from build123d import *

# Parameters (mm, degrees)
F0_W     = 18.5
F0_H     = 6.9
F0_H_2   = 6.8
F1_DEPTH = 3.25
F3_DEPTH = 1.5
F4_R     = 5
F6_D     = 4.4
F8_D     = 4.4


with BuildPart() as f1:
    # F0 (on Top) → F1 (new body)
    with BuildSketch(Plane.XY):
        with BuildLine():
            Line((-14.6952698517, 19.7279642442), (-29.6952698517, 19.7279642442))
            Line((-29.6952698517, 19.7279642442), (-41.8622746435, 10.5594685057))
            ThreePointArc((-41.8622746435, 10.5594685057), (-43.1340644308, 9.1283890545), (-43.7536388636, 7.3168799651))
            Line((-43.7536388636, 7.3168799651), (-43.7536388636, 6.0480798558))
            ThreePointArc((-43.7536388636, 6.0480798558), (-42.1412711242, 3.0324095441), (-38.9407541854, 1.8279642442))
            Line((-38.9407541854, 1.8279642442), (-14.6952698517, 1.8279642442))
            Line((-14.6952698517, 1.8279642442), (-14.6952698517, 3.0279642442))
            Line((-14.6952698517, 3.0279642442), (-14.6952698517, 9.8279642442))
            Line((-14.6952698517, 9.8279642442), (-14.6952698517, 11.8279642442))
            Line((-14.6952698517, 11.8279642442), (-14.6952698517, 18.7279642442))
            Line((-14.6952698517, 18.7279642442), (-14.6952698517, 19.7279642442))
        make_face()
        with BuildLine():
            ThreePointArc((-35.8858862752, 5.3242355882), (-39.5438948337, 7.153269317), (-37.7352474887, 10.8214004184))
            Line((-37.7352474887, 10.8214004184), (-33.8307472386, 12.0875827919))
            ThreePointArc((-33.8307472386, 12.0875827919), (-33.1317830892, 12.5942209035), (-32.8564297306, 13.4123978931))
            Line((-32.8564297306, 13.4123978931), (-32.8562668471, 13.7279642442))
            ThreePointArc((-32.8562668471, 13.7279642442), (-29.9562668471, 16.6279642442), (-27.0562668471, 13.7279642442))
            Line((-27.0562668471, 13.7279642442), (-27.0562668471, 10.3279642442))
            ThreePointArc((-27.0562668471, 10.3279642442), (-27.5890997188, 8.6388139758), (-29.0068091948, 7.5770986937))
            Line((-29.0068091948, 7.5770986937), (-35.8858862752, 5.3242355882))
        make_face(mode=Mode.SUBTRACT)
        with Locations((-5.4452698517, 15.2779642442)):
            Rectangle(F0_W, F0_H)
        with BuildLine():
            Line((-43.7536388636, 6.0480798558), (-43.7536388636, 7.3168799651))
            ThreePointArc((-43.7536388636, 7.3168799651), (-43.784850924, 7.0003621876), (-43.7952698517, 6.6824799105))
            ThreePointArc((-43.7952698517, 6.6824799105), (-43.784850924, 6.3645976333), (-43.7536388636, 6.0480798558))
        make_face()
        with Locations((-5.4452698517, 6.4279642442)):
            Rectangle(F0_W, F0_H_2)
    extrude(amount=F1_DEPTH)

    # F2 (on face) → F3 (join)
    with BuildSketch(Plane.XY.offset(3.25)):
        with BuildLine():
            Line((-14.6952698517, 18.7279642442), (-14.6952698517, 19.7279642442))
            Line((-14.6952698517, 19.7279642442), (-29.6952698517, 19.7279642442))
            Line((-29.6952698517, 19.7279642442), (-41.8622746435, 10.5594685057))
            ThreePointArc((-41.8622746435, 10.5594685057), (-43.5444062264, 5.142119485), (-38.9407541854, 1.8279642442))
            Line((-38.9407541854, 1.8279642442), (-14.6952698517, 1.8279642442))
            Line((-14.6952698517, 1.8279642442), (-14.6952698517, 3.0279642442))
            Line((-14.6952698517, 3.0279642442), (-14.6952698517, 9.8279642442))
            Line((-14.6952698517, 9.8279642442), (-14.6952698517, 11.8279642442))
            Line((-14.6952698517, 11.8279642442), (-14.6952698517, 18.7279642442))
        make_face()
        with BuildLine():
            ThreePointArc((-27.0562668471, 10.3279642442), (-27.5890997188, 8.6388139758), (-29.0068091948, 7.5770986937))
            Line((-29.0068091948, 7.5770986937), (-35.8858862752, 5.3242355882))
            ThreePointArc((-35.8858862752, 5.3242355882), (-39.5438948337, 7.153269317), (-37.7352474887, 10.8214004184))
            Line((-37.7352474887, 10.8214004184), (-33.8307472386, 12.0875827919))
            ThreePointArc((-33.8307472386, 12.0875827919), (-33.1317830892, 12.5942209035), (-32.8564297306, 13.4123978931))
            Line((-32.8564297306, 13.4123978931), (-32.8562668471, 13.7279642442))
            ThreePointArc((-32.8562668471, 13.7279642442), (-29.9562668471, 16.6279642442), (-27.0562668471, 13.7279642442))
            Line((-27.0562668471, 13.7279642442), (-27.0562668471, 10.3279642442))
        make_face(mode=Mode.SUBTRACT)
    extrude(amount=F3_DEPTH)

    # F4
    f4_edges = [f1.edges().sort_by_distance(p)[0] for p in [
        (-29.69527, 19.727964, 2.375),
    ]]
    fillet(f4_edges, radius=F4_R)

    # F6 (through all)
    with Locations(Plane.XY.offset(3.25)):
        with Locations((-7.6952698517, 15.7279642442)):
            Hole(F6_D / 2)

    # F8 (through all)
    with Locations(Plane.XY.offset(3.25)):
        with Locations((-10.3952698517, 6.2279642442)):
            Hole(F8_D / 2)


solid = f1.part
Build history of the part. All positions in model axes, mm. A direction names the side the tool comes from. Round coordinates to 2 decimals unless told otherwise and drop trailing zeros. Loops run counter-clockwise (first coordinate to the right, second up) from the corner with the lowest first, then second, coordinate; pieces in that order, holes last. Notation, with made-up numbers: (35, 61.25) -> (50, 61.25) arc R28 cw to (50, 91.25) -> close; hole circle Ø1 at (78.5, 33). An arc over 180 degrees is marked (long way). One line per item, written item: value. Start each with the question number.
Q1. Cut at C-C on y = 4.5. List the corners of the cut face in (x, z), plus the area to 3 significant figures.
Q2. Cut at B-B on z = 3.85. List the corners of the cut face in (x, y), plus the area to 4 significant figures.
Q3. Drop flat-ended pins along their axis: pin 1 Ø2.5 at (x, z) = (-8, 2.5) entering from +Y; pin 2 Ø7.5 at (x, y) = (-1.5, 16) entering from +Z; pin 3 Ø1 at (x, z) = (-3.5, 1) entering from -Y. Give the stop position or say it passes through.
Q4. Two-plate mould, pull along Y, no slides. Class faces 4 (the face through (-20, 11, 0)), 5 (the face through (-27.575, 8.659, 2.342)), 6 (the face through (-6, 18.728, 2)), 7 (the face through (-6, 3.028, 2)): released by +Y, released by -Y, zero draft, split by the parting line, or undercut.
Q5. Cut at A-A on x = -37. List the corners of the cut face in (y, z).
Q6. 3-axis set-ups, long thin cutter, end or side, ignore diameter. For faces 1 (the face through (-30.02, 16.627, 2.342)), 2 (the face through (-6, 6, 3.25)), 3 (the face through (-6, 9.828, 2)): which of +Z, -Z, +X, -X, +Y, -Y reach the whole face in a straight line?
Q7. Probe line 1 along Y through (x, z) = (-4, 3.15); line 2 along X through (y, z) = (13.75, 1.9); line 3 along X through (y, z) = (15.5, 3). List the from-to ranges inside material, lowest first.
Q8. Cut at D-D on x = -7. List the corners of the cut face in (y, z), plus the area to 3 significant figures.
Computed:
1. outline: (-43.28, 0) -> (-11.76, 0) -> (-11.76, 3.25) -> (-14.7, 3.25) -> (-14.7, 4.75) -> (-43.28, 4.75) -> close; (-9.03, 0) -> (3.8, 0) -> (3.8, 3.25) -> (-9.03, 3.25) -> close
1. area: 187 mm²
2. outline: (-41.86, 10.56) arc R4.85 ccw to (-38.94, 1.83) -> (-14.7, 1.83) -> (-14.7, 19.73) -> (-28.02, 19.73) arc R5 ccw to (-31.03, 18.72) -> close; hole (-37.74, 10.82) arc R2.9 ccw to (-35.89, 5.32) -> (-29.01, 7.58) arc R2.89 ccw to (-27.06, 10.33) -> (-27.06, 13.73) arc R2.9 ccw to (-32.86, 13.73) -> (-32.86, 13.41) arc R1.42 cw to (-33.83, 12.09) -> close
2. area: 352.5 mm²
3. pin 1: y = 18.73
3. pin 2: z = 3.25
3. pin 3: y = 3.03
4. face 4: zero draft
4. face 5: undercut
4. face 6: released by +Y
4. face 7: released by -Y
5. outline: (1.83, 0) -> (5.19, 0) -> (5.19, 4.75) -> (1.83, 4.75) -> close; (11.06, 0) -> (14.22, 0) -> (14.22, 4.75) -> (11.06, 4.75) -> close
6. face 1: +Z, -Z
6. face 2: +Z, +X, +Y, -Y
6. face 3: +Z, -Z, +X
7. line 1: 3.03 to 9.83, 11.83 to 18.73
7. line 2: -37.63 to -32.86, -27.06 to -8.66, -6.73 to 3.8
7. line 3: -35.31 to -32.25, -27.66 to -9.88, -5.51 to 3.8
8. outline: (3.03, 0) -> (9.83, 0) -> (9.83, 3.25) -> (3.03, 3.25) -> close; (11.83, 0) -> (13.64, 0) -> (13.64, 3.25) -> (11.83, 3.25) -> close; (17.82, 0) -> (18.73, 0) -> (18.73, 3.25) -> (17.82, 3.25) -> close
8. area: 31.0 mm²
